Check sheet for the drawn part. Datum: minimum x, y, z corner. Units: mm. Give positions to 0.01 mm unless a question says otherwise; leave off trailing zeros. Loops run counter-clockwise (first coordinate to the right, second up) from the corner with the lowest first, then second, coordinate; pieces in that order, holes last. Notation, with made-up numbers: (-22, 24) - (-10, 24) arc R23 ccw to (-10, 61) - close; hole circle Ø10 at (11, 31). An arc over 180 degrees is marked (long way). One line per item, written item: value. Start each with the question number.
1. Sectioned sample at A-A (y = 42.75). Record the cut outline in (x, z), plus the area to 3 significant figures.
2. Scan lines: L1, parallel to Y at x = 31, z = 0.7; L2, parallel to Y at x = 29.5, z = 1.65; L3, parallel to X at y = 43.5, z = 1.65. Record each from-to range of solid material in increasing order. Write a range as [from, to].
3. Sectioned sample at C-C (z = 1.1). Record the cut outline in (x, y), plus the area to 3 significant figures.
4. Sectioned sample at B-B (x = 31). Record the cut outline in (y, z), plus the area to 3 significant figures.
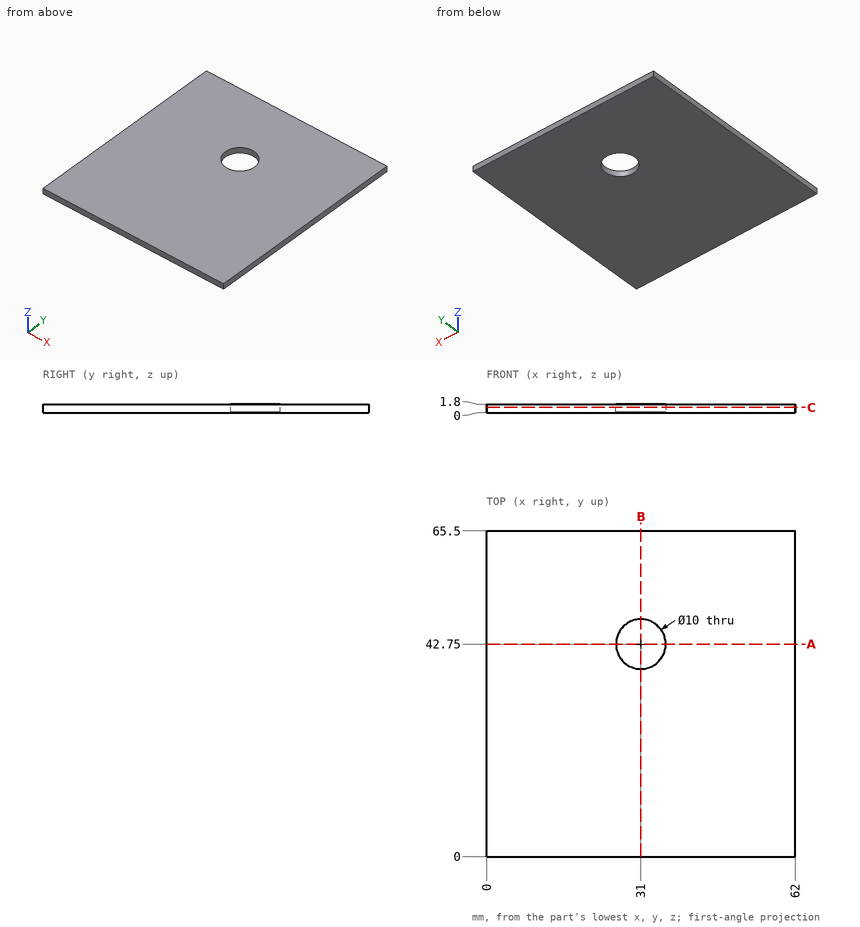
Results are:
1. outline: (0, 0) - (26, 0) - (26, 1.8) - (0, 1.8) - close; (36, 0) - (62, 0) - (62, 1.8) - (36, 1.8) - close
1. area: 93.6 mm^2
2. L1: y = [0, 37.75], [47.75, 65.5]
2. L2: y = [0, 37.98], [47.52, 65.5]
2. L3: x = [0, 26.06], [35.94, 62]
3. outline: (0, 0) - (62, 0) - (62, 65.5) - (0, 65.5) - close; hole circle Ø10 at (31, 42.75)
3. area: 3,980 mm^2
4. outline: (0, 0) - (37.75, 0) - (37.75, 1.8) - (0, 1.8) - close; (47.75, 0) - (65.5, 0) - (65.5, 1.8) - (47.75, 1.8) - close
4. area: 99.9 mm^2
